from build123d import *

# Parameters (mm, degrees)
F1_DEPTH = 10
F2_DEPTH = 17
F3_W     = 100
F3_H     = 35
F4_DEPTH = 3
F5_SIZE2 = 99.99999
F5_SIZE  = 7.49999
F6_R     = 8
F8_DEPTH = 7
F9_W     = 5.1550631039
F9_H     = 7


# Not quite as in the source:
# - a fillet or chamfer is up to 0.001 mm smaller than in the source, because OpenCascade refuses the exact size


with BuildPart() as f1:
    # F0 (on Top) → F1 (new body)
    with BuildSketch(Plane.XY):
        Polygon((-58.5, -8.5), (-58.5, -2.5), (-58.5, 0), (-58.5, 2.5), (-58.5, 8.5), (-63.5, 0), align=None)
        Polygon((-58.5, -2.5), (-55, -2.5), (-55, 2.5), (-58.5, 2.5), (-58.5, 0), align=None)
    extrude(amount=F1_DEPTH)

    # F0 (on Top) → F2 (join)
    with BuildSketch(Plane.XY):
        Polygon((-55, -17.5), (55, -17.5), (55, 17.5), (-55, 17.5), (-55, 2.5), (-55, -2.5), align=None)
    extrude(amount=F2_DEPTH)

    # F3 (on face) → F4 (join)
    with BuildSketch(Plane.XY.offset(17)):
        with Locations((5, 0)):
            Rectangle(F3_W, F3_H)
    extrude(amount=F4_DEPTH)

    # F5 (size 7.5 and 100 in the source; OpenCascade refuses exactly that, so slightly less here)
    f5_edges = [f1.edges().sort_by_distance(p)[0] for p in [
        (55, -17.5, 10),
        (55, 17.5, 10),
    ]]
    f5_side = f1.faces().sort_by_distance((55, 0, 10))[0]
    chamfer(f5_edges, length=F5_SIZE, length2=F5_SIZE2, reference=f5_side)

    # F6
    f6_edges = [f1.edges().sort_by_distance(p)[0] for p in [
        (55, -10.00001, 10),
        (55, 10.00001, 10),
    ]]
    fillet(f6_edges, radius=F6_R)

    # F7 (on face) → F8 (join)
    with BuildSketch(Plane.XY):
        with BuildLine():
            ThreePointArc((118.6121593217, 42.5), (89.7807277981, 72.2473973087), (50.3125, 84.8338219329))
            ThreePointArc((50.3125, 84.8338219329), (46.5767340156, 83.4879420476), (45, 79.8435971134))
            Line((45, 79.8435971134), (45, 0))
            Line((45, 0), (50, 2.8867513459))
            Line((50, 2.8867513459), (50, 74.3303437366))
            ThreePointArc((50, 74.3303437366), (51.708597057, 78.0942070001), (55.6666666667, 79.2856999857))
            ThreePointArc((55.6666666667, 79.2856999857), (89.5397594579, 66.4545696505), (114.2820323028, 40))
            Line((114.2820323028, 40), (118.6121593217, 42.5))
        make_face()
        with BuildLine():
            ThreePointArc((120.9846922835, 38.0962798523), (119.8308271392, 40.3155963576), (118.6121593217, 42.5))
            Line((118.6121593217, 42.5), (114.2820323028, 40))
            ThreePointArc((114.2820323028, 40), (115.4987732023, 37.8143223789), (116.6465834297, 35.5916715378))
            Line((116.6465834297, 35.5916715378), (120.9846922835, 38.0962798523))
        make_face()
        with BuildLine():
            ThreePointArc((120.9846922835, -38.0962798523), (130, 0), (120.9846922835, 38.0962798523))
            Line((120.9846922835, 38.0962798523), (116.6465834297, 35.5916715378))
            ThreePointArc((116.6465834297, 35.5916715378), (125, 0), (116.6465834297, -35.5916715378))
            Line((116.6465834297, -35.5916715378), (120.9846922835, -38.0962798523))
        make_face()
        with BuildLine():
            Line((50, -2.8867513459), (45, 0))
            Line((45, 0), (45, -79.8435971134))
            ThreePointArc((45, -79.8435971134), (46.5767340156, -83.4879420476), (50.3125, -84.8338219329))
            ThreePointArc((50.3125, -84.8338219329), (89.7807277981, -72.2473973087), (118.6121593217, -42.5))
            Line((118.6121593217, -42.5), (114.2820323028, -40))
            ThreePointArc((114.2820323028, -40), (89.5397594579, -66.4545696505), (55.6666666667, -79.2856999857))
            ThreePointArc((55.6666666667, -79.2856999857), (51.708597057, -78.0942070001), (50, -74.3303437366))
            Line((50, -74.3303437366), (50, -2.8867513459))
        make_face()
        Polygon((50, 2.8867513459), (45, 0), (50, -2.8867513459), align=None)
        with BuildLine():
            ThreePointArc((118.6121593217, -42.5), (119.8308271392, -40.3155963576), (120.9846922835, -38.0962798523))
            Line((120.9846922835, -38.0962798523), (116.6465834297, -35.5916715378))
            ThreePointArc((116.6465834297, -35.5916715378), (115.4987732023, -37.8143223789), (114.2820323028, -40))
            Line((114.2820323028, -40), (118.6121593217, -42.5))
        make_face()
    extrude(amount=F8_DEPTH)

    # F9 (on face) → F10 (join, up to the next surface of F1)
    with BuildSketch(Plane.YZ.offset(55)):
        with Locations((0, 3.5)):
            Rectangle(F9_W, F9_H)
    extrude(until=Until.NEXT)


solid = f1.part
Could you check a few things on this model? Use its own coordinates, in mm. A direction names the side the tool comes from. Give positions to 0.01 mm unless a question says otherwise; leave off trailing zeros. Loops run counter-clockwise (first coordinate to the right, second up) from the corner with the lowest first, then second, coordinate; pieces in that order, holes last. Notation, with made-up numbers: (43, -31) -> (50, -31) arc R24 cw to (50, -2) -> close; hole circle Ø2 at (-30, 29.25). An arc over 180 degrees is marked (long way). Return JSON: item names as keys, results as strings.
Item 1: If we section it at B-B on y = -6: List the corners of the cut face in (x, z) for me.
Geometry results:
{"outline": "(-59.97, 0) -> (-58.5, 0) -> (-58.5, 10) -> (-59.97, 10) -> close; (-55, 0) -> (54.23, 0) -> (54.23, 20) -> (-45, 20) -> (-45, 17) -> (-55, 17) -> close; (124.77, 0) -> (129.79, 0) -> (129.79, 7) -> (124.77, 7) -> close"}
Item 2: If we section it at C-C on z = 12.25: List the corners of the cut face in (x, y) for me, plus the area to 3 significant figures.
Geometry results:
{"outline": "(-55, -17.5) -> (-45, -17.5) -> (47.6, -10.56) arc R8 ccw to (55, -2.58) -> (55, 2.58) arc R8 ccw to (47.6, 10.56) -> (-45, 17.5) -> (-55, 17.5) -> close", "area": "3,080 mm²"}
Item 3: Which directions (+Z, -Z, +X, -X, +Y, -Y) give clear straight access to the entire face, cutting with the end or side of a thin tool? Please do faces 1 (the flat face through (-50, 17.5, 8)), 2 (the flat face through (78, 0, 7)), 3 (the flat face through (4, 0, 20)), 4 (the cylindrical face through (51.66, 78.05, 3.45)), 5 (the cylindrical face through (52.92, 7.96, 9.86)).
Geometry results:
{"face 1": "+Z, -Z, -X, +Y", "face 2": "+Z, +X", "face 3": "+Z, +X, -X, +Y, -Y", "face 4": "+Z, -Z", "face 5": "+Z"}
Item 4: I need wall thicknesses on L1, parallel to Z at x = 47.5, y = 47; L2, parallel to X at y = 25, z = 3.5; L3, parallel to X at y = 67.5, z = 1. Which ranges of each line are inside material? Lowest first, please. Write a range as from..to.
Geometry results:
{"L1": "z = 0..7", "L2": "x = 45..50, 120.99..126.24", "L3": "x = 45..50, 87.94..96.66"}
Item 5: We'd pull the mould along Y, two halves only. Please class faces 6 (the flat face through (-58.5, 5, 5)), 7 (the cylindrical face through (46.62, 83.53, 3.45)), 8 (the cylindrical face through (52.807, -8.08, 10.14)): +Y half, -Y half, draft (parallel to the pull), parting line (faces both ways), or undercut.
Geometry results:
{"face 6": "draft", "face 7": "+Y half", "face 8": "undercut"}
Item 6: If we section it at A-A on x = 83: List the corners of the cut face in (y, z) for me, plus the area to 3 significant figures.
Geometry results:
{"outline": "(-76.03, 0) -> (-70.4, 0) -> (-70.4, 7) -> (-76.03, 7) -> close; (-2.58, 0) -> (2.58, 0) -> (2.58, 7) -> (-2.58, 7) -> close; (70.4, 0) -> (76.03, 0) -> (76.03, 7) -> (70.4, 7) -> close", "area": "115 mm²"}
Item 7: If we section it at D-D on y = -69.5: List the corners of the cut face in (x, z) for me, plus the area to 3 significant figures.
Geometry results:
{"outline": "(45, 0) -> (50, 0) -> (50, 7) -> (45, 7) -> close; (84.62, 0) -> (93.94, 0) -> (93.94, 7) -> (84.62, 7) -> close", "area": "100 mm²"}
Item 8: I'm going to push flat-ended pins straight in: pin 1 (2 mm diameter, centred on x = 75, z = 4, fed in from -Y); pin 2 (10 mm diameter, centred on x = -30, z = 4.5, fed in from -Y); pin 3 (7.5 mm diameter, centred on y = -31.5, z = 3.5, fed in from -X); pin 4 (12 mm diameter, centred on x = 18, y = -16, fed in from +Z). Where does each tip first touch, or does it pass through?
Geometry results:
{"pin 1": "stops at y = -79.9", "pin 2": "stops at y = -16.75", "pin 3": "stops at x = 45", "pin 4": "stops at z = 20"}
